Input: part model. Units: mm. Frame: model coordinates. Face numbers are marked on the shaded views. A direction names the side the tool comes from. Give positions to 0.01 mm unless a question says otherwise; leave off trailing zeros. Write each loop counter-clockwise with the first axis right and the second up, starting at its lowest first coordinate (ties: lowest second). Pieces come first, ordered by that corner, then holes. Notation, with made-up numbers: (27, 8) - (40, 8) arc R10 ccw to (40, 25) - close; hole circle Ø4 at (-1, 44). An arc over 180 degrees is marked (long way). Answer as CSV lines item,"result".
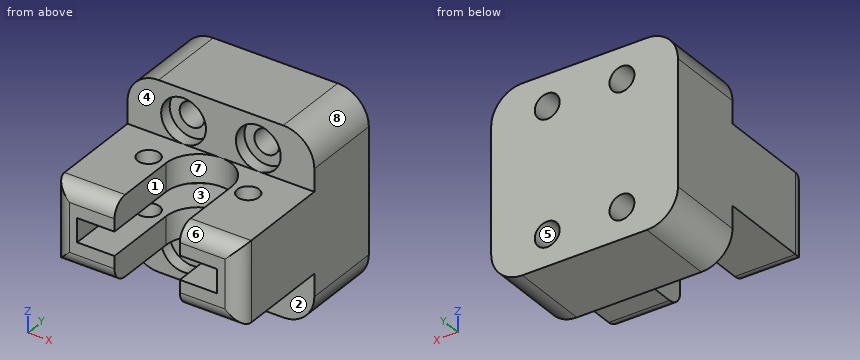
```python
from build123d import *

# Parameters (mm, degrees)
SKETCH2_W               = 30
SKETCH2_H               = 30
BOSS_EXTRUDE1_DEPTH     = 30
CUT_EXTRUDE1_REACH      = 47
SKETCH3_R               = 1.75
CUT_EXTRUDE2_START      = -15
SKETCH4_R               = 1.75
CUT_EXTRUDE2_DEPTH      = 1.9
CUT_EXTRUDE2_DEPTH_BACK = 1.9
CUT_EXTRUDE3_REACH      = 38.742
SKETCH5_R               = 2
SKETCH6_W               = 30
SKETCH6_H               = 8.6
CUT_EXTRUDE5_DEPTH      = 17.25
SKETCH8_R               = 3.6
CUT_EXTRUDE6_DEPTH      = 2
FILLET1_R               = 5
FILLET2_R               = 2.5


with BuildPart() as part:
    # Sketch2 → Boss-Extrude1 (new body)
    with BuildSketch(Plane(origin=(0, 0, 0), x_dir=(1, 0, 0), z_dir=(0, 1, 0))):
        Rectangle(SKETCH2_W, SKETCH2_H)
    extrude(amount=BOSS_EXTRUDE1_DEPTH)

    # Sketch3 → Cut-Extrude1 (cut, up to next)
    with BuildSketch(Plane.XY.offset(15), mode=Mode.PRIVATE) as cut_extrude1_sk1:
        with Locations((-8, 12)):
            Circle(SKETCH3_R)
    cut_extrude1_tool1 = extrude(cut_extrude1_sk1.sketch, amount=-CUT_EXTRUDE1_REACH, mode=Mode.PRIVATE) & part.part
    # Sketch3 → Cut-Extrude1 (cut, up to next)
    with BuildSketch(Plane.XY.offset(15), mode=Mode.PRIVATE) as cut_extrude1_sk2:
        with Locations((8, 12)):
            Circle(SKETCH3_R)
    cut_extrude1_tool2 = extrude(cut_extrude1_sk2.sketch, amount=-CUT_EXTRUDE1_REACH, mode=Mode.PRIVATE) & part.part
    # Sketch3 → Cut-Extrude1 (cut, up to next)
    with BuildSketch(Plane.XY.offset(15), mode=Mode.PRIVATE) as cut_extrude1_sk3:
        with BuildLine():
            ThreePointArc((5.25, 12), (0, 17.25), (-5.25, 12))
            Line((-5.25, 12), (5.25, 12))
        make_face()
    cut_extrude1_tool3 = extrude(cut_extrude1_sk3.sketch, amount=-CUT_EXTRUDE1_REACH, mode=Mode.PRIVATE) & part.part
    # Sketch3 → Cut-Extrude1 (cut, up to next)
    with BuildSketch(Plane.XY.offset(15), mode=Mode.PRIVATE) as cut_extrude1_sk4:
        with BuildLine():
            Line((5.25, 12), (-5.25, 12))
            ThreePointArc((-5.25, 12), (0, 6.75), (5.25, 12))
        make_face()
    cut_extrude1_tool4 = extrude(cut_extrude1_sk4.sketch, amount=-CUT_EXTRUDE1_REACH, mode=Mode.PRIVATE) & part.part
    # Sketch3 → Cut-Extrude1 (cut, up to next)
    with BuildSketch(Plane.XY.offset(15), mode=Mode.PRIVATE) as cut_extrude1_sk5:
        with BuildLine():
            ThreePointArc((5.25, 12), (0, 17.25), (-5.25, 12))
            Line((-5.25, 12), (5.25, 12))
        make_face()
    cut_extrude1_tool5 = extrude(cut_extrude1_sk5.sketch, amount=-CUT_EXTRUDE1_REACH, mode=Mode.PRIVATE) & part.part
    # Sketch3 → Cut-Extrude1 (cut, up to next)
    with BuildSketch(Plane.XY.offset(15), mode=Mode.PRIVATE) as cut_extrude1_sk6:
        with BuildLine():
            Line((5.25, 12), (-5.25, 12))
            ThreePointArc((-5.25, 12), (0, 6.75), (5.25, 12))
        make_face()
    cut_extrude1_tool6 = extrude(cut_extrude1_sk6.sketch, amount=-CUT_EXTRUDE1_REACH, mode=Mode.PRIVATE) & part.part
    # Sketch3 → Cut-Extrude1 (cut, up to next)
    with BuildSketch(Plane.XY.offset(15), mode=Mode.PRIVATE) as cut_extrude1_sk7:
        with BuildLine():
            ThreePointArc((5.25, 12), (0, 6.75), (-5.25, 12))
            Line((-5.25, 12), (-5.25, 0))
            Line((-5.25, 0), (5.25, 0))
            Line((5.25, 0), (5.25, 12))
        make_face()
    cut_extrude1_tool7 = extrude(cut_extrude1_sk7.sketch, amount=-CUT_EXTRUDE1_REACH, mode=Mode.PRIVATE) & part.part
    add(cut_extrude1_tool1.solids().sort_by_distance((-8, 12, 15))[0], mode=Mode.SUBTRACT)
    add(cut_extrude1_tool2.solids().sort_by_distance((8, 12, 15))[0], mode=Mode.SUBTRACT)
    add(cut_extrude1_tool3.solids().sort_by_distance((0, 14.228169, 15))[0], mode=Mode.SUBTRACT)
    add(cut_extrude1_tool4.solids().sort_by_distance((0, 9.771831, 15))[0], mode=Mode.SUBTRACT)
    add(cut_extrude1_tool5.solids().sort_by_distance((0, 14.228169, 15))[0], mode=Mode.SUBTRACT)
    add(cut_extrude1_tool6.solids().sort_by_distance((0, 9.771831, 15))[0], mode=Mode.SUBTRACT)
    add(cut_extrude1_tool7.solids().sort_by_distance((0, 4.02549, 15))[0], mode=Mode.SUBTRACT)

    # Sketch4 → Cut-Extrude2 (cut, two sides)
    with BuildSketch(Plane.XY.offset(15).offset(CUT_EXTRUDE2_START)) as cut_extrude2_sk:
        with BuildLine():
            Line((-5.25, 0), (-5.25, 12))
            ThreePointArc((-5.25, 12), (0, 17.25), (5.25, 12))
            Line((5.25, 12), (5.25, 0))
            Line((5.25, 0), (11.25, 0))
            Line((11.25, 0), (11.25, 12))
            ThreePointArc((11.25, 12), (0, 23.25), (-11.25, 12))
            Line((-11.25, 12), (-11.25, 0))
            Line((-11.25, 0), (-5.25, 0))
        make_face()
        with Locations((8, 12)):
            Circle(SKETCH4_R, mode=Mode.SUBTRACT)
        with Locations((-8, 12)):
            Circle(SKETCH4_R, mode=Mode.SUBTRACT)
    extrude(amount=CUT_EXTRUDE2_DEPTH, mode=Mode.SUBTRACT)
    extrude(cut_extrude2_sk.sketch, amount=-CUT_EXTRUDE2_DEPTH_BACK, mode=Mode.SUBTRACT)

    # Sketch5 → Cut-Extrude3 (cut, up to next)
    with BuildSketch(Plane(origin=(0, 30, 0), x_dir=(1, 0, 0), z_dir=(0, 1, 0)), mode=Mode.PRIVATE) as cut_extrude3_sk1:
        with Locations(Location((-6, 10, 0), (0, 0, 270))):
            Circle(SKETCH5_R)
    cut_extrude3_tool1 = extrude(cut_extrude3_sk1.sketch, amount=-CUT_EXTRUDE3_REACH, mode=Mode.PRIVATE) & part.part
    # Sketch5 → Cut-Extrude3 (cut, up to next)
    with BuildSketch(Plane(origin=(0, 30, 0), x_dir=(1, 0, 0), z_dir=(0, 1, 0)), mode=Mode.PRIVATE) as cut_extrude3_sk2:
        with Locations(Location((6, 10, 0), (0, 0, 247.975687163))):
            Circle(SKETCH5_R)
    cut_extrude3_tool2 = extrude(cut_extrude3_sk2.sketch, amount=-CUT_EXTRUDE3_REACH, mode=Mode.PRIVATE) & part.part
    # Sketch5 → Cut-Extrude3 (cut, up to next)
    with BuildSketch(Plane(origin=(0, 30, 0), x_dir=(1, 0, 0), z_dir=(0, 1, 0)), mode=Mode.PRIVATE) as cut_extrude3_sk3:
        with Locations(Location((6, -10, 0), (0, 0, 270))):
            Circle(SKETCH5_R)
    cut_extrude3_tool3 = extrude(cut_extrude3_sk3.sketch, amount=-CUT_EXTRUDE3_REACH, mode=Mode.PRIVATE) & part.part
    # Sketch5 → Cut-Extrude3 (cut, up to next)
    with BuildSketch(Plane(origin=(0, 30, 0), x_dir=(1, 0, 0), z_dir=(0, 1, 0)), mode=Mode.PRIVATE) as cut_extrude3_sk4:
        with Locations(Location((-6, -10, 0), (0, 0, 292.024312837))):
            Circle(SKETCH5_R)
    cut_extrude3_tool4 = extrude(cut_extrude3_sk4.sketch, amount=-CUT_EXTRUDE3_REACH, mode=Mode.PRIVATE) & part.part
    add(cut_extrude3_tool1.solids().sort_by_distance((-6, 30, -10))[0], mode=Mode.SUBTRACT)
    add(cut_extrude3_tool2.solids().sort_by_distance((6, 30, -10))[0], mode=Mode.SUBTRACT)
    add(cut_extrude3_tool3.solids().sort_by_distance((6, 30, 10))[0], mode=Mode.SUBTRACT)
    add(cut_extrude3_tool4.solids().sort_by_distance((-6, 30, 10))[0], mode=Mode.SUBTRACT)

    # Sketch6 → Cut-Extrude5 (cut)
    with BuildSketch(Plane.XZ):
        with Locations((0, 10.7)):
            Rectangle(SKETCH6_W, SKETCH6_H)
        with Locations((0, -10.7)):
            Rectangle(SKETCH6_W, SKETCH6_H)
    extrude(amount=-CUT_EXTRUDE5_DEPTH, mode=Mode.SUBTRACT)

    # Sketch8 → Cut-Extrude6 (cut)
    with BuildSketch(Plane.XZ.offset(-17.25)):
        with Locations(Location((-6, 10, 0), (0, 0, 270))):
            Circle(SKETCH8_R)
        with Locations(Location((6, 10, 0), (0, 0, 270))):
            Circle(SKETCH8_R)
        with Locations(Location((6, -10, 0), (0, 0, 270))):
            Circle(SKETCH8_R)
        with Locations(Location((-6, -10, 0), (0, 0, 90))):
            Circle(SKETCH8_R)
    extrude(amount=-CUT_EXTRUDE6_DEPTH, mode=Mode.SUBTRACT)

    # Fillet1
    fillet1_edges = [part.edges().sort_by_distance(p)[0] for p in [
        (15, 23.625, 15),
        (-15, 23.625, 15),
        (-15, 23.625, -15),
        (15, 23.625, -15),
    ]]
    fillet(fillet1_edges, radius=FILLET1_R)

    # Fillet2
    fillet2_edges = [part.edges().sort_by_distance(p)[0] for p in [
        (-15, 0, 0),
        (15, 0, 0),
        (-10.125, 0, -6.4),
        (10.125, 0, -6.4),
        (-10.125, 0, 6.4),
        (10.125, 0, 6.4),
    ]]
    fillet(fillet2_edges, radius=FILLET2_R)


solid = part.part
```
Item 1: Cut plane C-C on x = 4.5. Return the cut outline in (y, z), plus the area to 3 significant figures.
The answers:
outline,"(14.7, -6.4) - (17.25, -6.4) - (17.25, -6.73) - (19.25, -6.73) - (19.25, -8.68) - (30, -8.68) - (30, 8.68) - (19.25, 8.68) - (19.25, 6.73) - (17.25, 6.73) - (17.25, 6.4) - (14.7, 6.4) - (14.7, 1.9) - (22.31, 1.9) - (22.31, -1.9) - (14.7, -1.9) - close; (17.25, -15) - (30, -15) - (30, -11.32) - (19.25, -11.32) - (19.25, -13.27) - (17.25, -13.27) - close; (17.25, 13.27) - (19.25, 13.27) - (19.25, 11.32) - (30, 11.32) - (30, 15) - (17.25, 15) - close"
area,"303 mm²"
Item 2: Cut plane D-D on y = 13.25. Count the separate pieces of the cut face and the enclosed holes in it, plus the area to 3 significant figures.
The answers:
separate pieces,"6"
enclosed holes,"0"
area,"163 mm²"
Item 3: Cut plane A-A on z = -3.25. Return the cut outline in (x, y), plus the area to 3 significant figures.
The answers:
outline,"(-15, 2.5) arc R2.5 ccw to (-12.5, 0) - (-5.25, 0) - (-5.25, 12) arc R5.25 cw to (5.25, 12) - (5.25, 0) - (12.5, 0) arc R2.5 ccw to (15, 2.5) - (15, 30) - (-15, 30) - close; hole circle Ø3.5 at (-8, 12); hole circle Ø3.5 at (8, 12)"
area,"709 mm²"
Item 4: Ray query, line 1 (X direction, y = 25, z = 10); line 2 (Z direction, x = -5.75, y = 5.5); line 3 (X direction, y = 18, z = -9.75). Return the intervals inside material, ascending. Write a range as from..to.
The answers:
line 1,"-15..-8, -4..4, 8..15"
line 2,"-6.4..-1.9, 1.9..6.4"
line 3,"-15..-9.59, -2.41..2.41, 9.59..15"
Item 5: Contact query for flat-ended pins moving along their axis: pin 1 (2.5 mm diameter, centred on x = 1, z = 12, fed in from -Y); pin 2 (3.5 mm diameter, centred on x = 6, z = 10, fed in from +Y); pin 3 (4.5 mm diameter, centred on x = -10, y = 6.5, fed in from +Z); pin 4 (6 mm diameter, centred on y = 5, z = -6.5, fed in from +X). Output: stop coordinate, or through.
The answers:
pin 1,"y = 17.25"
pin 2,"through"
pin 3,"z = 6.4"
pin 4,"x = 15"
Item 6: Reachability of the marked faces 1, 2, 3 and 4 from +Z, -Z, +X, -X, +Y, -Y: full face, straight path, thin tool, end or side. Return the list, or none.
The answers:
face 1,"+Z, -Z, -Y"
face 2,"-Z, +X, -X, -Y"
face 3,"-Y"
face 4,"+Z, +X, -X, -Y"
Item 7: Cut plane B-B on y = 9.25. Return the cut outline in (x, z).
The answers:
outline,"(-15, -6.4) - (-5.25, -6.4) - (-5.25, -1.9) - (-11.25, -1.9) - (-11.25, 1.9) - (-5.25, 1.9) - (-5.25, 6.4) - (-15, 6.4) - close; (5.25, -6.4) - (15, -6.4) - (15, 6.4) - (5.25, 6.4) - (5.25, 1.9) - (11.25, 1.9) - (11.25, -1.9) - (5.25, -1.9) - close"
Item 8: Mould query, pull axis X, two halves, no side actions, for the marked faces 5, 6, 7 and 8. Classes: +X half, -X half, draft (parallel to the pull), parting line (faces both ways), or undercut.
The answers:
face 5,"undercut"
face 6,"draft"
face 7,"undercut"
face 8,"+X half"
